from build123d import *

# Parameters (mm, degrees)
SKETCH_R  = 2.775
PAD_DEPTH = 2


with BuildPart() as part:
    # Sketch → Pad (new body)
    with BuildSketch(Plane.XZ):
        with BuildLine():
            Line((0, 0), (58.956405, 0))
            Line((58.956405, 0), (50.807402, 8.149004))
            ThreePointArc((56.447133, 12.2955), (35.051339, 35.487738), (50.807402, 8.149004))
            Line((68.27, 0.472633), (56.447133, 12.2955))
            Line((68.27, 0.472633), (68.27, 44.45))
            Line((68.27, 44.45), (0, 44.45))
            Line((0, 44.45), (0, 0))
        make_face()
        with Locations((7.94, 6.35)):
            Circle(SKETCH_R, mode=Mode.SUBTRACT)
        with Locations((7.94, 38.1)):
            Circle(SKETCH_R, mode=Mode.SUBTRACT)
    extrude(amount=PAD_DEPTH)


solid = part.part
Could you check a few things on this model? Use its own coordinates, in mm. A direction names the side the tool comes from. Give positions to 0.01 mm unless a question says otherwise; leave off trailing zeros. Order: outer loops, then holes, each group sorted by start corner. A loop starts at its lowest first (then second) coordinate and runs counter-clockwise, first axis right, second up. Notation, with made-up numbers: (-36, -27) - (15, -27) arc R9 cw to (15, -21) - close; hole circle Ø4 at (0, 53.25). An arc over 180 degrees is marked (long way). One line per item, written item: value. Start each with the question number.
1. If I drill on probe 1 along Z at (x, y) = (7.94, -1.6) (3 decimals); probe 2 along X at (y, z) = (-1.2, 21); probe 3 along X at (y, z) = (-1.6, 12), over which ranges is the centre line in solid material (lowest first)?
2. Imagine slicing it at C-C on z = 32. List the corners of the cut face in (x, y) for me, plus the area to 3 significant figures.
3. Thinking about a two-plate mould opening in X: for faces 3 (the face through (29, -1, 0)), 4 (the face through (54.939, -0.986, 4.017)), 5 (the face through (68.27, -1, 22)), which applies, +X half, -X half, draft (parallel to the pull), parting line (faces both ways), or undercut?
4. For faces 1 (the face through (62.44, -0.99, 6.3)), 2 (the face through (0, -1, 23)), which set-ups out of +Z, -Z, +X, -X, +Y, -Y let a thin tool reach every point of the face, with its end or its side?
5. Imagine slicing it at B-B on x = 7.94. List the corners of the cut face in (y, z) for me (3 decimals).
6. Imagine slicing it at A-A on y = -1.65. Give the number of separate pieces and of enclosed holes in the cut face, plus the area to 3 significant figures.
7. Imagine slicing it at D-D on x = 44. List the corners of the cut face in (y, z) for me.
Values:
1. probe 1: 0 to 3.575, 9.125 to 35.325, 40.875 to 44.45
1. probe 2: 0 to 28.67, 60.24 to 68.27
1. probe 3: 0 to 32.73, 56.74 to 68.27
2. outline: (0, -2) - (31.59, -2) - (31.59, 0) - (0, 0) - close; (57.32, -2) - (68.27, -2) - (68.27, 0) - (57.32, 0) - close
2. area: 85.1 mm²
3. face 3: draft
3. face 4: undercut
3. face 5: +X half
4. face 1: +Y, -Y
4. face 2: +Z, -Z, -X, +Y, -Y
5. outline: (-2, 0) - (0, 0) - (0, 3.575) - (-2, 3.575) - close; (-2, 9.125) - (0, 9.125) - (0, 35.325) - (-2, 35.325) - close; (-2, 40.875) - (0, 40.875) - (0, 44.45) - (-2, 44.45) - close
6. separate pieces: 1
6. enclosed holes: 2
6. area: 2,100 mm²
7. outline: (-2, 0) - (0, 0) - (0, 6.83) - (-2, 6.83) - close; (-2, 38.57) - (0, 38.57) - (0, 44.45) - (-2, 44.45) - close
